Design review of the part built by this model. Coordinates are the model's own, in mm. Face numbers are marked on the shaded views. A direction names the side the tool comes from. Round coordinates to 2 decimals unless told otherwise and drop trailing zeros. Loops run counter-clockwise (first coordinate to the right, second up) from the corner with the lowest first, then second, coordinate; pieces in that order, holes last. Notation, with made-up numbers: M 47,71 L 68,71 A32 cw 68,103 Z; hole C 29.25,-18 d11. An arc over 180 degrees is marked long. One line per item, written item: value. Start each with the question number.
Item 1: We need section B-B (y = 0). Write out the cut boundary in (x, z).
Item 2: Mouldability with a two-part tool opening along Y and no side actions: class the marked faces 6, 7 and 8 as released by +Y, released by -Y, zero draft, split by the parting line, or undercut.
Item 3: We need section D-D (y = 9). Write out the cut boundary in (x, z) (3 decimals).
Item 4: We need section C-C (x = -18.5). Write out the cut boundary in (y, z) (3 decimals).
Item 5: Clearance check with flat-ended pins moving along their axes: pin 1 (0.8 mm diameter, centred on x = 0.5, z = -0.5, fed in from +Y); pin 2 (1.5 mm diameter, centred on x = 13.5, z = -1, fed in from +Y); pin 3 (2 mm diameter, centred on y = 12.5, z = 0, fed in from +X). State where each tip first meets the part, or that it passes through.
Item 6: For line 1 along Y through (x, z) = (19.5, 0) (3 decimals); line 2 along Z through (x, y) = (0, 14) (3 decimals); line 3 along Y through (x, z) = (0, -3.2), list the stretches that pass through material, from the lowest coordinate up.
Item 7: For the marked faces 1, 2, 3, 4 and 5, list the 3-axis set-ups (+Z, -Z, +X, -X, +Y, -Y) from which the entire face can be reached by the end or side of a thin tool; tool diameter is ignored.
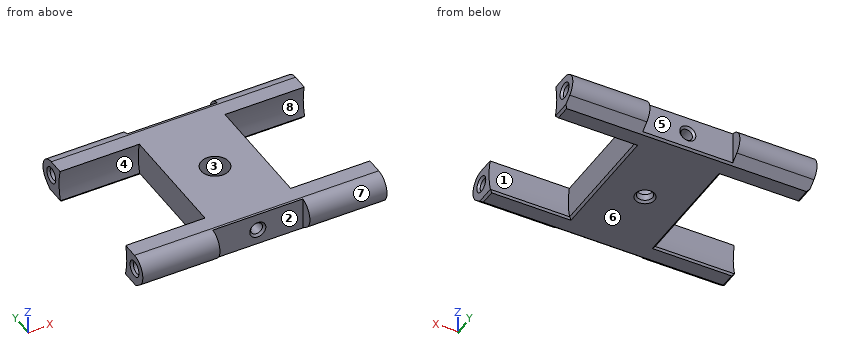
from build123d import *

# Parameters (mm, degrees)
PAD_DEPTH           = 28.5
SKETCH001_R         = 14.25
POCKET_DEPTH        = 18.5
SKETCH002_R         = 1.375
POCKET001_DEPTH     = 12
SKETCH003_W         = 4
SKETCH003_H         = 10.5
POCKET002_DEPTH     = 8
SKETCH004_R         = 1.75
POCKET003_DEPTH     = 8
SKETCH005_R         = 3.25
POCKET004_DEPTH     = 6
SKETCH006_R         = 1.375
POCKET005_DEPTH     = 10
SKETCH007_R         = 1.375
POCKET006_DEPTH     = 10
CHAMFER_SIZE        = 0.5
CHAMFER001_SIZE     = 0.5
CLONE001_ROLL_ANGLE = -90


with BuildPart() as recess_pocket:
    # Sketch → Pad (new body)
    with BuildSketch(Plane.YZ):
        with BuildLine():
            ThreePointArc((2.722222, 19.699888), (-1.166667, 20.799832), (-3.5, 17.5))
            Line((-3.5, 17.5), (-3.5, -17.5))
            ThreePointArc((-3.5, -17.5), (-1.166657, -20.799835), (2.722235, -19.699872))
            Line((2.722235, -19.699872), (4.5, -17.5))
            Line((4.5, 17.5), (4.5, -17.5))
            Line((4.5, 17.5), (2.722222, 19.699888))
        make_face()
    extrude(amount=PAD_DEPTH)

    # Sketch001 → Pocket (cut)
    with BuildSketch(Plane.YZ.offset(28.5)):
        Circle(SKETCH001_R)
    extrude(amount=-POCKET_DEPTH, mode=Mode.SUBTRACT)

    # Sketch002 → Pocket001 (cut)
    with BuildSketch(Plane.YZ.offset(28.5)):
        with Locations((0, -17.5)):
            Circle(SKETCH002_R)
        with Locations((0, 17.5)):
            Circle(SKETCH002_R)
    extrude(amount=-POCKET001_DEPTH, mode=Mode.SUBTRACT)

    # Sketch003 → Pocket002 (cut)
    with BuildSketch(Plane(origin=(0, -3.5, 0), x_dir=(0, 0, -1), z_dir=(0, -1, 0))):
        with Locations((-20, 5.25)):
            Rectangle(SKETCH003_W, SKETCH003_H)
        with Locations((20, 5.25)):
            Rectangle(SKETCH003_W, SKETCH003_H)
    extrude(amount=-POCKET002_DEPTH, mode=Mode.SUBTRACT)


with BuildPart() as motor_bracket_printing:
    # Part__Mirroring: instance of recess-pocket
    add(recess_pocket.part.mirror(Plane(origin=(0, 0, 0), x_dir=(0, -1, 0), z_dir=(1, 0, 0))))

    # Fusion: union recess-pocket
    add(recess_pocket.part)

    # Sketch004 → Pocket003 (cut)
    with BuildSketch(Plane.XZ.offset(3.5)):
        Circle(SKETCH004_R)
    extrude(amount=-POCKET003_DEPTH, mode=Mode.SUBTRACT)

    # Sketch005 → Pocket004 (cut)
    with BuildSketch(Plane.XZ.offset(3.5)):
        Circle(SKETCH005_R)
    extrude(amount=-POCKET004_DEPTH, mode=Mode.SUBTRACT)

    # Sketch006 → Pocket005 (cut)
    with BuildSketch(Plane.XY.offset(18)):
        with Locations((0, 0.5)):
            Circle(SKETCH006_R)
    extrude(amount=-POCKET005_DEPTH, mode=Mode.SUBTRACT)

    # Sketch007 → Pocket006 (cut)
    with BuildSketch(Plane(origin=(0, 0, -18), x_dir=(1, 0, 0), z_dir=(0, 0, -1))):
        with Locations((0, -0.5)):
            Circle(SKETCH007_R)
    extrude(amount=-POCKET006_DEPTH, mode=Mode.SUBTRACT)

    # Chamfer
    chamfer_edges = [motor_bracket_printing.edges().sort_by_distance(p)[0] for p in [
        (28.5, -1.375, -17.5),
        (-28.5, -1.375, -17.5),
        (-28.5, -1.375, 17.5),
        (28.5, -1.375, 17.5),
        (-1.375, 0.5, -18),
        (-1.375, 0.5, 18),
    ]]
    chamfer(chamfer_edges, length=CHAMFER_SIZE)

    # Chamfer001
    chamfer001_edges = [motor_bracket_printing.edges().sort_by_distance(p)[0] for p in [
        (28.5, 4.5, -15.510409),
        (19.25, 4.5, -13.520817),
        (-10, 4.5, 0),
        (-19.25, 4.5, -13.520817),
        (-19.25, 4.5, 13.520817),
        (-28.5, 4.5, -15.510409),
        (-28.5, 4.5, 15.510409),
        (28.5, 4.5, 15.510409),
        (19.25, 4.5, 13.520817),
        (10, 4.5, 0),
        (-1.75, 4.5, 0),
    ]]
    chamfer(chamfer001_edges, length=CHAMFER001_SIZE)


with BuildPart() as motor_bracket_printing_1:
    # Clone001 roll: moved
    add(motor_bracket_printing.part.rotate(Axis((0, 0, 0), (1, 0, 0)), CLONE001_ROLL_ANGLE))


with BuildPart() as motor_bracket_printing_2:
    # Clone001 placement: moved
    add(motor_bracket_printing_1.part)


solid = motor_bracket_printing_2.part
A:
1. outline: M -10,-4 L -9.5,-4.5 L -2.25,-4.5 L -1.75,-4 L -1.75,-2.5 L -3.25,-2.5 L -3.25,3.5 L -10,3.5 Z; M 1.75,-4 L 2.25,-4.5 L 9.5,-4.5 L 10,-4 L 10,3.5 L 3.25,3.5 L 3.25,-2.5 L 1.75,-2.5 Z
2. face 6: zero draft
2. face 7: released by -Y
2. face 8: undercut
3. outline: M -10,-4 L -9.5,-4.5 L 9.5,-4.5 L 10,-4 L 10,3.5 L -10,3.5 Z; hole C 0,-0.5 d2.75
4. outline: M -19.7,-2.722 L -17.5,-4.5 L -14.021,-4.5 L -13.67,-4.023 A14.25 cw -13.813,3.5 L -17.5,3.5 A3.5 ccw Z; M 13.67,-4.023 L 14.021,-4.5 L 17.5,-4.5 L 19.7,-2.722 A3.5 ccw 17.5,3.5 L 13.813,3.5 A14.25 cw Z; hole C -17.5,0 d2.75; hole C 17.5,0 d2.75
5. pin 1: y = 8
5. pin 2: y = 20.99
5. pin 3: x = 10
6. line 1: -21 to -18.875, -16.125 to -14.25, 14.25 to 16.125, 18.875 to 21
6. line 2: -4.5 to -1.875, 0.875 to 3.5
6. line 3: -18 to -1.75, 1.75 to 18
7. face 1: +X
7. face 2: +Z, -Z, -Y
7. face 3: +Z
7. face 4: -X
7. face 5: +Z, -Z, +Y
